Verification items for the finished model (mm, model axes). Face numbers are marked on the shaded views. A direction names the side the tool comes from. Round coordinates to 2 decimals unless told otherwise and drop trailing zeros. Order: outer loops, then holes, each group sorted by start corner. A loop starts at its lowest first (then second) coordinate and runs counter-clockwise, first axis right, second up. Notation, with made-up numbers: (4, 40) -> (17, 40) arc R32 ccw to (17, 78) -> close; hole circle Ø5 at (55, -29). An arc over 180 degrees is marked (long way). Return JSON: item names as keys, results as strings. Group by question number.
1) Section check B-B on x = -1.75. Enter the section's corners in (y, z).
2) Section check C-C on z = -6.75. Enter the section's corners in (x, y).
3) Section check A-A on y = -18. Enter the section's corners in (x, z) (3 decimals), plus the area to 3 significant figures.
4) Draft check along X on the marked faces 1, 2 and 3. Enter one of: pulls with the +X half, pulls with the -X half, needs draft (parallel to the pull), parting line crosses it, or undercut.
5) Depth check by flat-ended pin: pin 1 (6 mm diameter, centred on y = -9, z = 4, fed in from +X); pin 2 (1 mm diameter, centred on x = 5, y = -10.5, fed in from -Z) (3 decimals); pin 3 (4 mm diameter, centred on y = -20.5, z = -4, fed in from -X). Enter the tip coordinate at first touch or a pass-through.
6) Tool access check on the marked faces 4 and 5. Record the directions out of +Z, -Z, +X, -X, +Y, -Y that give a thin tool (end or side, any length) a straight path to the whole face; none if there is none.
7) Scan lines: L1, parallel to Z at x = 8.75, y = -12.5; L2, parallel to Z at x = 0.25, y = -13.75; L3, parallel to X at y = -20.5, z = -2. Record each from-to range of solid material in increasing order.
```python
from build123d import *

# Parameters (mm, degrees)
F0_R     = 9.525
F1_DEPTH = 25.4
F3_DEPTH = 25.401
F4_DEPTH = 11.0998
F6_DEPTH = 25.4


with BuildPart() as f1:
    # F0 (on Front) → F1 (new body)
    with BuildSketch(Plane.XZ):
        with Locations((-1e-06, -3e-06)):
            Circle(F0_R)
    extrude(amount=F1_DEPTH)

    # F2 (on Front) → F3 (cut, through all)
    with BuildSketch(Plane.XZ):
        with BuildLine():
            Line((-1.107965, 4.707283), (-4.835918, 4.707283))
            Line((-4.835918, 4.707283), (-4.835918, 0))
            ThreePointArc((-4.835918, 0), (-3.791051, 3.002339), (-1.107965, 4.707283))
        make_face()
    extrude(amount=F3_DEPTH, mode=Mode.SUBTRACT)

    # F2 (on Front) → F4 (cut)
    with BuildSketch(Plane.XZ):
        with BuildLine():
            Line((-1.107965, 4.707283), (-4.835918, 4.707283))
            Line((-4.835918, 4.707283), (-4.835918, 0))
            ThreePointArc((-4.835918, 0), (-3.791051, 3.002339), (-1.107965, 4.707283))
        make_face()
        with BuildLine():
            ThreePointArc((1.107965, 4.707283), (0, 4.835918), (-1.107965, 4.707283))
            Line((-1.107965, 4.707283), (1.107965, 4.707283))
        make_face()
        with BuildLine():
            ThreePointArc((-0.41918, -4.817717), (-3.564634, -3.267949), (-4.835918, 0))
            Line((-4.835918, 0), (-4.835918, -4.817717))
            Line((-4.835918, -4.817717), (-0.41918, -4.817717))
        make_face()
        with BuildLine():
            Line((4.689082, 4.707283), (1.107965, 4.707283))
            ThreePointArc((1.107965, 4.707283), (3.392231, 3.446574), (4.689082, 1.182631))
            Line((4.689082, 1.182631), (4.689082, 4.707283))
        make_face()
        with BuildLine():
            Line((0.41918, -4.817717), (-0.41918, -4.817717))
            ThreePointArc((-0.41918, -4.817717), (0, -4.835918), (0.41918, -4.817717))
        make_face()
        with BuildLine():
            ThreePointArc((4.835918, 0), (4.799069, 0.595856), (4.689082, 1.182631))
            Line((4.689082, 1.182631), (4.689082, -1.182631))
            ThreePointArc((4.689082, -1.182631), (4.799069, -0.595856), (4.835918, 0))
        make_face()
        with BuildLine():
            ThreePointArc((4.689082, -1.182631), (3.134812, -3.682263), (0.41918, -4.817717))
            Line((0.41918, -4.817717), (4.689082, -4.817717))
            Line((4.689082, -4.817717), (4.689082, -1.182631))
        make_face()
    extrude(amount=F4_DEPTH, mode=Mode.SUBTRACT)

    # F5 (on face) → F6 (cut)
    with BuildSketch(Plane.XZ.offset(25.4)):
        Polygon((4.445, 7.698966), (-4.445, 7.698966), (-8.89, 0), (-4.445, -7.698966), (4.445, -7.698966), (8.89, 0), align=None)
        with BuildLine():
            ThreePointArc((-1.107965, 4.707283), (-3.791051, 3.002339), (-4.835918, 0))
            Line((-4.835918, 0), (-4.835918, 4.707283))
            Line((-4.835918, 4.707283), (-1.107965, 4.707283))
        make_face(mode=Mode.SUBTRACT)
    extrude(amount=-F6_DEPTH, mode=Mode.SUBTRACT)


solid = f1.part
```
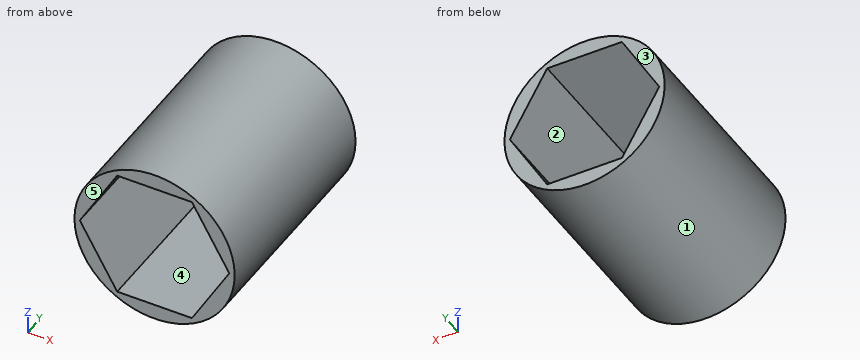
Check result:
{
 "1": {"outline": "(-25.4, -9.36) -> (0, -9.36) -> (0, -7.7) -> (-25.4, -7.7) -> close; (-25.4, 7.7) -> (0, 7.7) -> (0, 9.36) -> (-25.4, 9.36) -> close"},
 "2": {"outline": "(-6.72, -25.4) -> (-4.99, -25.4) -> (-4.99, 0) -> (-6.72, 0) -> close; (4.99, -25.4) -> (6.72, -25.4) -> (6.72, 0) -> (4.99, 0) -> close"},
 "3": {"outline": "circle Ø19.05 at (0, 0); hole (-8.89, 0) -> (-4.445, -7.699) -> (4.445, -7.699) -> (8.89, 0) -> (4.445, 7.699) -> (-4.445, 7.699) -> close", "area": "79.7 mm^2"},
 "4": {"face 1": "parting line crosses it", "face 2": "undercut", "face 3": "needs draft"},
 "5": {"pin 1": "x = 9.47", "pin 2": "z = -8.395", "pin 3": "x = -9.31"},
 "6": {"face 4": "+Y, -Y", "face 5": "+Z, -Z, +X, -X, -Y"},
 "7": {"L1": "-3.76 to -0.24, 0.24 to 3.76", "L2": "-9.52 to -7.7, 7.7 to 9.52", "L3": "-9.31 to -7.74, 7.74 to 9.31"}
}
